```python
from build123d import *

# Parameters (mm, degrees)
SKETCH1_W           = 24.429357143
SKETCH1_H           = 3.175
SKETCH1_W_2         = 24.429357142
SKETCH1_W_3         = 3.175
SKETCH1_H_2         = 12.7
BOSS_EXTRUDE1_DEPTH = 6.35
SKETCH2_R           = 1.499997
SKETCH2_R_2         = 1.5
SKETCH2_W           = 12.7
SKETCH2_H           = 3.175
SKETCH2_W_2         = 3.175
SKETCH2_H_2         = 12.7
CUT_EXTRUDE1_DEPTH  = 7.35
SKETCH3_W           = 171.0055
SKETCH3_H           = 101.6
SKETCH3_H_2         = 44.45
CUT_EXTRUDE2_DEPTH  = 7.35


with BuildPart() as part:
    # Sketch1 → Boss-Extrude1 (new body)
    with BuildSketch(Plane(origin=(0, 0, 0), x_dir=(1, 0, 0), z_dir=(0, 1, 0))):
        Polygon((0, 174.625), (0, 95.25), (-3.175, 95.25), (-3.175, 85.725), (0, 85.725), (0, 73.025), (-3.175, 73.025), (-3.175, 60.325), (0, 60.325), (0, 47.625), (-3.175, 47.625), (-3.175, 34.925), (0, 34.925), (0, 22.225), (-3.175, 22.225), (-3.175, 9.525), (0, 9.525), (0, -3.175), (-3.175, -3.175), (-3.175, -15.875), (0, -15.875), (0, -28.575), (-3.175, -28.575), (-3.175, -38.1), (0, -38.1), (0, -174.625), (171.0055, -174.625), (171.0055, 174.625), align=None)
        with Locations((36.644035714, -39.6875)):
            Rectangle(SKETCH1_W, SKETCH1_H, mode=Mode.SUBTRACT)
        with Locations((85.50275, -39.6875)):
            Rectangle(SKETCH1_W_2, SKETCH1_H, mode=Mode.SUBTRACT)
        Polygon((122.146785714, -38.1), (142.4305, -38.1), (142.4305, -28.575), (145.6055, -28.575), (145.6055, -38.1), (146.576142857, -38.1), (146.576142857, -41.275), (122.146785714, -41.275), align=None, mode=Mode.SUBTRACT)
        with Locations((144.018, -9.525)):
            Rectangle(SKETCH1_W_3, SKETCH1_H_2, mode=Mode.SUBTRACT)
        with Locations((144.018, 15.875)):
            Rectangle(SKETCH1_W_3, SKETCH1_H_2, mode=Mode.SUBTRACT)
        with Locations((144.018, 41.275)):
            Rectangle(SKETCH1_W_3, SKETCH1_H_2, mode=Mode.SUBTRACT)
        with Locations((144.018, 66.675)):
            Rectangle(SKETCH1_W_3, SKETCH1_H_2, mode=Mode.SUBTRACT)
        Polygon((142.4305, 85.725), (142.4305, 95.25), (122.146785714, 95.25), (122.146785714, 98.425), (146.576142857, 98.425), (146.576142857, 95.25), (145.6055, 95.25), (145.6055, 85.725), align=None, mode=Mode.SUBTRACT)
        with Locations((85.50275, 96.8375)):
            Rectangle(SKETCH1_W_2, SKETCH1_H, mode=Mode.SUBTRACT)
        with Locations((36.644035714, 96.8375)):
            Rectangle(SKETCH1_W, SKETCH1_H, mode=Mode.SUBTRACT)
    extrude(amount=BOSS_EXTRUDE1_DEPTH)

    # Sketch2 → Cut-Extrude1 (cut, through all)
    with BuildSketch(Plane(origin=(0, 6.35, 0), x_dir=(1, 0, 0), z_dir=(0, 1, 0))):
        with Locations((9.525, -165.1)):
            Circle(SKETCH2_R)
        with Locations((9.525, 165.1)):
            Circle(SKETCH2_R)
        with Locations((22.225, -53.975)):
            Circle(SKETCH2_R_2)
        with Locations((22.225, 111.125)):
            Circle(SKETCH2_R_2)
        with Locations((158.790821429, -42.8625)):
            Rectangle(SKETCH2_W, SKETCH2_H)
        with Locations((158.790821429, 100.0125)):
            Rectangle(SKETCH2_W, SKETCH2_H)
        with Locations((7.9375, -53.975)):
            Rectangle(SKETCH2_W_2, SKETCH2_H_2)
        with Locations((7.9375, 111.125)):
            Rectangle(SKETCH2_W_2, SKETCH2_H_2)
    extrude(amount=-CUT_EXTRUDE1_DEPTH, mode=Mode.SUBTRACT)

    # Sketch3 → Cut-Extrude2 (cut, through all)
    with BuildSketch(Plane(origin=(0, 6.35, 0), x_dir=(1, 0, 0), z_dir=(0, 1, 0))):
        with Locations((85.50275, -123.825)):
            Rectangle(SKETCH3_W, SKETCH3_H)
        with Locations((85.50275, 152.4)):
            Rectangle(SKETCH3_W, SKETCH3_H_2)
    extrude(amount=-CUT_EXTRUDE2_DEPTH, mode=Mode.SUBTRACT)


solid = part.part
```
Verification items for the finished model (mm, model axes). A direction names the side the tool comes from. Round coordinates to 2 decimals unless told otherwise and drop trailing zeros. Order: outer loops, then holes, each group sorted by start corner. A loop starts at its lowest first (then second) coordinate and runs counter-clockwise, first axis right, second up. Notation, with made-up numbers: (3.25, -6) -> (28.25, -6) arc R23 cw to (28.25, 2) -> close; hole circle Ø11 at (-33, 75.5). An arc over 180 degrees is marked (long way). Put each result on its own line as item: value. Start each with the question number.
(1) Material ranges on line 1 along Z through (x, y) = (154, 5.25) (3 decimals); line 2 along Z through (x, y) = (35, 4.5) (3 decimals); line 3 along X through (y, z) = (1.75, -89.5) (1 decimal), recorded low to high.
(2) Tool access check on faces 1 (the face through (0, 3, -3)), 2 (the face through (9.525, 3, -111)), 3 (the face through (-3.175, 3, -16)). Record the directions out of +Z, -Z, +X, -X, +Y, -Y that give a thin tool (end or side, any length) a straight path to the whole face; none if there is none.
(3) Section check A-A (x = 128). Enter the section's corners in (y, z) (3 decimals), then the cut area to 3 significant figures.
(4) Draft check along Z on faces 4 (the face through (135, 3, 41.275)), 5 (the face through (84, 3, -130.175)), 6 (the face through (-3.175, 3, 33)), 7 (the face through (85, 3, -98.425)). Enter one of: +Z half, -Z half, draft (parallel to the pull), parting line (faces both ways), or undercut.
(5) Section check C-C (y = 1.5). State how many separate pieces and enclosed holes the cut face has, then the cut area to 3 significant figures.
(6) Depth check by flat-ended pin: pin 1 Ø1 at (x, y) = (-1, 2.5) entering from +Z. Enter the tip coordinate at first touch or a pass-through.
Completed:
1. line 1: z = -130.175 to -101.6, -98.425 to 41.275, 44.45 to 73.025
1. line 2: z = -130.175 to -98.425, -95.25 to 38.1, 41.275 to 73.025
1. line 3: x = -3.2 to 142.4, 145.6 to 171
2. face 1: -X, +Y, -Y
2. face 2: +Y, -Y
2. face 3: +Z, -Z, -X, +Y, -Y
3. outline: (0, -130.175) -> (6.35, -130.175) -> (6.35, -98.425) -> (0, -98.425) -> close; (0, -95.25) -> (6.35, -95.25) -> (6.35, 38.1) -> (0, 38.1) -> close; (0, 41.275) -> (6.35, 41.275) -> (6.35, 73.025) -> (0, 73.025) -> close
3. area: 1,250 mm2
4. face 4: undercut
4. face 5: -Z half
4. face 6: draft
4. face 7: undercut
5. separate pieces: 1
5. enclosed holes: 16
5. area: 34,100 mm2
6. pin 1: stops at z = 38.1
